```python
from build123d import *

# Parameters (mm, degrees)
F1_DEPTH       = 32
F2_W           = 10
F2_H           = 20
F3_DEPTH       = 50.001
F5_D           = 4.2
F5_DEPTH       = 34.15
F5_CBORE_D     = 9.75
F5_CBORE_DEPTH = 5
F5_TIP         = 1.2618073
F7_D           = 4.2
F9_D           = 5.5
F9_CBORE_D     = 9.75
F9_CBORE_DEPTH = 5
F10_R          = 2.5
F11_DEPTH      = 7


with BuildPart() as f1:
    # F0 (on Top) → F1 (new body)
    with BuildSketch(Plane.XY):
        with BuildLine():
            ThreePointArc((7.5, -14.1332940251), (-8.2623874884, 13.7015675377), (9, -13.2287565553))
            Line((9, -13.2287565553), (9, -23.749))
            Line((9, -23.749), (23, -23.749))
            Line((23, -23.749), (23, 0))
            ThreePointArc((23, 0), (17.5842402782, 14.8254677444), (3.8874353183, 22.6690945264))
            Line((3.8874353183, 22.6690945264), (-17, 26.251))
            Line((-17, 26.251), (-27, 26.251))
            Line((-27, 26.251), (-27, -23.749))
            Line((-27, -23.749), (7.5, -23.749))
            Line((7.5, -23.749), (7.5, -14.1332940251))
        make_face()
    extrude(amount=F1_DEPTH)

    # F2 (on face) → F3 (cut, through all)
    with BuildSketch(Plane.XZ.offset(23.749)):
        with Locations((-22, 16)):
            Rectangle(F2_W, F2_H)
    extrude(amount=-F3_DEPTH, mode=Mode.SUBTRACT)

    # F5
    with Locations(Plane.YZ.offset(23)):
        with Locations((-18.7706, 16)):
            CounterBoreHole(F5_D / 2, F5_CBORE_D / 2, F5_CBORE_DEPTH, depth=F5_DEPTH)
            with Locations((0, 0, -(F5_DEPTH + F5_TIP / 2))):  # 118° drill point
                Cone(0, F5_D / 2, F5_TIP, mode=Mode.SUBTRACT)

    # F7 (through all)
    with Locations(Plane.XY.offset(32)):
        with Locations((-22, 18), (-22, 0), (-22, -18)):
            Hole(F7_D / 2)

    # F9 (through all)
    with Locations(Plane.XY.offset(32)):
        with Locations((-12.1156, 19.8332124892)):
            CounterBoreHole(F9_D / 2, F9_CBORE_D / 2, F9_CBORE_DEPTH)

    # F10 (on face) → F11 (cut)
    with BuildSketch(Plane(origin=(0, 0, 0), x_dir=(1, 0, 0), z_dir=(0, 0, -1))):
        with Locations((-12.1156, -19.8332124892)):
            Circle(F10_R)
    extrude(amount=-F11_DEPTH, mode=Mode.SUBTRACT)


solid = f1.part
```
Geometry check sheet. Reference: the model listing, model coordinates, mm. A direction names the side the tool comes from. Give positions to 0.01 mm unless a question says otherwise; leave off trailing zeros. Loops run counter-clockwise (first coordinate to the right, second up) from the corner with the lowest first, then second, coordinate; pieces in that order, holes last. Notation, with made-up numbers: M 38.5,67 L 88.5,67 A10 cw 88.5,76 Z; hole C 82.25,4 d3. An arc over 180 degrees is marked long. Write item = value, one per line. Start each with the question number.
1. Tool access check on faces 1 (the face through (17.73, 14.65, 15.78)), 2 (the face through (7.5, -21.1, 15.8)), 3 (the face through (-17, 1, 16)), 4 (the face through (-1.96, -19.9, 17.77)). Record the directions out of +Z, -Z, +X, -X, +Y, -Y that give a thin tool (end or side, any length) a straight path to the whole face; none if there is none.
2. Section check A-A, the plane x = -22. Give the number of separate pieces and of enclosed holes in the cut face, plus the area to 3 significant figures.
3. Draft check along Y on faces 5 (the face through (-27, 2, 3)), 6 (the face through (-23.13, -16.23, 2.96)), 7 (the face through (-6.41, 24.435, 15.776)). Enter one of: +Y half, -Y half, draft (parallel to the pull), parting line (faces both ways), or undercut.
4. Go/stop test with flat-tipped pins: P1, Ø5, axis at y = -18.77, z = 16, coming from the +X side; P2, Ø6, axis at y = 5.5, z = 13.5, coming from the -X side; P3, Ø2, axis at x = -12, z = 14.5, coming from the +Y side; P4, Ø2.5, axis at x = -22, y = 0, coming from the +Z side. Record where each tip stops, or that it passes through.
5. Section check C-C, the plane x = -10. Enter the section's corners in (y, z), plus the area to 3 significant figures.
6. Section check B-B, the plane y = 18. Enter the section's corners in (x, z), plus the area to 3 significant figures.
7. Thickness scan on probe 1 along Y at (x, z) = (-22, 2); probe 2 along Y at (x, z) = (-2.25, 16); probe 3 along Y at (x, z) = (-13.5, 9). Record the ranges inside material, lowest first.
8. Section check D-D, the plane x = -3.5. Enter the section's corners in (y, z), plus the area to 3 significant figures.
Values follow:
q1.face_1 = +Z, -Z, +X, +Y
q1.face_2 = +Z, -Z, -Y
q1.face_3 = -X, +Y, -Y
q1.face_4 = +X
q2.separate_pieces = 8
q2.enclosed_holes = 0
q2.area = 449 mm^2
q3.face_5 = draft
q3.face_6 = undercut
q3.face_7 = +Y half
q4.P1 = 18
q4.P2 = -17
q4.P3 = 25.57
q4.P4 = through
q5.outline = M -23.75,0 L -12.49,0 L -12.49,32 L -23.75,32 Z; M 12.49,0 L 18.08,0 L 18.08,27 L 15.44,27 L 15.44,32 L 12.49,32 Z; M 21.59,0 L 25.05,0 L 25.05,32 L 24.23,32 L 24.23,27 L 21.59,27 Z; hole C -18.77,16 d4.2
q5.area = 610 mm^2
q6.outline = M -27,0 L -24.1,0 L -24.1,6 L -27,6 Z; M -27,26 L -24.1,26 L -24.1,32 L -27,32 Z; M -19.9,0 L -14.17,0 L -14.17,27 L -16.63,27 L -16.63,32 L -19.9,32 L -19.9,26 L -17,26 L -17,6 L -19.9,6 Z; M -10.07,0 L 14.32,0 L 14.32,32 L -7.6,32 L -7.6,27 L -10.07,27 Z
q6.area = 916 mm^2
q7.probe_1 = -23.75 to -20.1, -15.9 to -2.1, 2.1 to 15.9, 20.1 to 26.25
q7.probe_2 = -23.75 to -20.87, -16.67 to -15.84, 15.84 to 23.72
q7.probe_3 = -23.75 to -8.59, 8.59 to 17.46, 22.21 to 25.65
q8.outline = M -23.75,0 L -15.61,0 L -15.61,32 L -23.75,32 Z; M 15.61,0 L 23.94,0 L 23.94,32 L 15.61,32 Z; hole C -18.77,16 d4.2
q8.area = 513 mm^2
